Model file for the job. Use its own axes, mm. A direction names the side the tool comes from. Coordinates: 2 decimals unless noted, no trailing zeros. Order: outer loops, then holes, each group sorted by start corner. A loop starts at its lowest first (then second) coordinate and runs counter-clockwise, first axis right, second up. Notation, with made-up numbers: (-19, 55) -> (30, 55) arc R19 cw to (30, 74) -> close; hole circle Ø3 at (-6.5, 21). An arc over 180 degrees is marked (long way). Return JSON: item names as keys, results as strings. Group by question number.
1) Flat gauge pins, fed straight in: pin 1 (1.1 mm diameter, centred on x = 0, y = -0.5, fed in from +Z); pin 2 (1 mm diameter, centred on x = 1, z = -4.5, fed in from +Y); pin 3 (3 mm diameter, centred on y = -2, z = -4, fed in from -X). Where does each tip first touch, or does it go through?
2) Probe line 1 (Y direction, x = 0.05, z = -1.25); line 2 (Z direction, x = -0.75, y = -0.5); line 3 (Z direction, x = -1.5, y = -1.25). List the from-to ranges inside material, lowest first.
3) Cut at A-A (z = 1.25). Write the cut outline in (x, y), and give its area (3 significant figures).
4) Pull direction X, two halves, no side cores. Call faces 1 (the flat face through (2, 0, 2)), 2 (the flat face through (0, 0, 0.5)), 3 (the cylindrical face through (-0.596, 2.685, 0.99)): +X half, -X half, draft (parallel to the pull), parting line (faces both ways), or undercut.
5) Which spindle directions (+Z, -Z, +X, -X, +Y, -Y) get a long thin tool onto all of the face, cutting with end or side? Do faces 4 (the flat face through (0, 0, -8)), 5 (the cylindrical face through (1.5, -0.07, -3.85)), 6 (the flat face through (-0.63, 1.08, 1.26)). Say none if no direction does.
6) Cut at C-C (z = -6). Write the cut outline in (x, y), and give its area (3 significant figures).
7) Cut at B-B (y = 0). Write the cut outline in (x, z).
Autodesk Inventor part; units mm, degrees
ref_plane "YZ Plane" through (0, 0, 0) normal (1, 0, 0) x (0, 1, 0)
ref_plane "XZ Plane" through (0, 0, 0) normal (0, 1, 0) x (-1, 0, 0)
ref_plane "XY Plane" through (0, 0, 0) normal (0, 0, 1) x (1, 0, 0)
sketch "スケッチ1" plane through (0, 0, 0) normal (0, 0, 1) x (1, 0, 0)
  circle A0 centre (0, 0) radius 2.75
  dimension "d0" = 5.5
extrude "押し出し1" add sketch "スケッチ1" along normal blind 2
sketch "スケッチ2" plane through (0, 0, 0) normal (0, 0, -1) x (-1, 0, 0)
  circle A0 centre (0, 0) radius 2.75
  circle A1 centre (0, 0) radius 1.5
  dimension "d3" = 3
extrude "押し出し2" add sketch "スケッチ2" along normal blind 8 contours A1
sketch "スケッチ3" plane through (0, 0, 2) normal (0, 0, 1) x (1, 0, 0)
  circle A0 centre (0, 0) radius 2.75
  line L0 (0, 1.4434) -> (1.25, 0.7217)
  line L1 (1.25, 0.7217) -> (1.25, -0.7217)
  line L2 (1.25, -0.7217) -> (0, -1.4434)
  line L3 (0, -1.4434) -> (-1.25, -0.7217)
  line L4 (-1.25, -0.7217) -> (-1.25, 0.7217)
  line L5 (-1.25, 0.7217) -> (0, 1.4434)
  dimension "d6" = 1.25
extrude "押し出し3" cut sketch "スケッチ3" against normal blind 1.5 contours L0 L1 L2 L3 L4 L5
fillet "フィレット1" radius 0.3 2 edges at (-2.75, 0, 2) (-2.75, 0, 0)
fillet "フィレット2" radius 0.2 19 edges at (-0.625, 1.0825, 2) (-1.25, 0, 2) (-0.625, -1.0825, 2) (0.625, -1.0825, 2) (1.25, 0, 2) (0.625, 1.0825, 2) (-0.625, 1.0825, 0.5) (0.625, 1.0825, 0.5) (0, 1.4434, 1.25) (-1.25, 0.7217, 1.25) (-0.625, -1.0825, 0.5) (-1.25, -0.7217, 1.25) (-1.25, 0, 0.5) (1.25, 0, 0.5) (1.25, 0.7217, 1.25) (1.25, -0.7217, 1.25) (0.625, -1.0825, 0.5) (0, -1.4434, 1.25) (1.5, 0, -8)
thread "ねじ2"
Answers below:
{
 "1": {"pin 1": "stops at z = 0.5", "pin 2": "stops at y = 1.41", "pin 3": "stops at x = -1.41"},
 "2": {"line 1": "y = -1.5 to 1.5", "line 2": "z = -8 to 0.5", "line 3": "z = 0 to 2"},
 "3": {"outline": "circle Ø5.5 at (0, 0); hole (-1.25, -0.61) arc R0.2 ccw to (-1.15, -0.78) -> (-0.1, -1.39) arc R0.2 ccw to (0.1, -1.39) -> (1.15, -0.78) arc R0.2 ccw to (1.25, -0.61) -> (1.25, 0.61) arc R0.2 ccw to (1.15, 0.78) -> (0.1, 1.39) arc R0.2 ccw to (-0.1, 1.39) -> (-1.15, 0.78) arc R0.2 ccw to (-1.25, 0.61) -> close", "area": "18.4 mm^2"},
 "4": {"face 1": "draft", "face 2": "undercut", "face 3": "parting line"},
 "5": {"face 4": "-Z, +X, -X, +Y, -Y", "face 5": "-Z", "face 6": "+Z"},
 "6": {"outline": "circle Ø3 at (0, 0)", "area": "7.07 mm^2"},
 "7": {"outline": "(-2.75, 0.3) arc R0.3 ccw to (-2.45, 0) -> (-1.5, 0) -> (-1.5, -7.8) arc R0.2 ccw to (-1.3, -8) -> (1.3, -8) arc R0.2 ccw to (1.5, -7.8) -> (1.5, 0) -> (2.45, 0) arc R0.3 ccw to (2.75, 0.3) -> (2.75, 1.7) arc R0.3 ccw to (2.45, 2) -> (1.45, 2) arc R0.2 ccw to (1.25, 1.8) -> (1.25, 0.7) arc R0.2 cw to (1.05, 0.5) -> (-1.05, 0.5) arc R0.2 cw to (-1.25, 0.7) -> (-1.25, 1.8) arc R0.2 ccw to (-1.45, 2) -> (-2.45, 2) arc R0.3 ccw to (-2.75, 1.7) -> close"}
}
